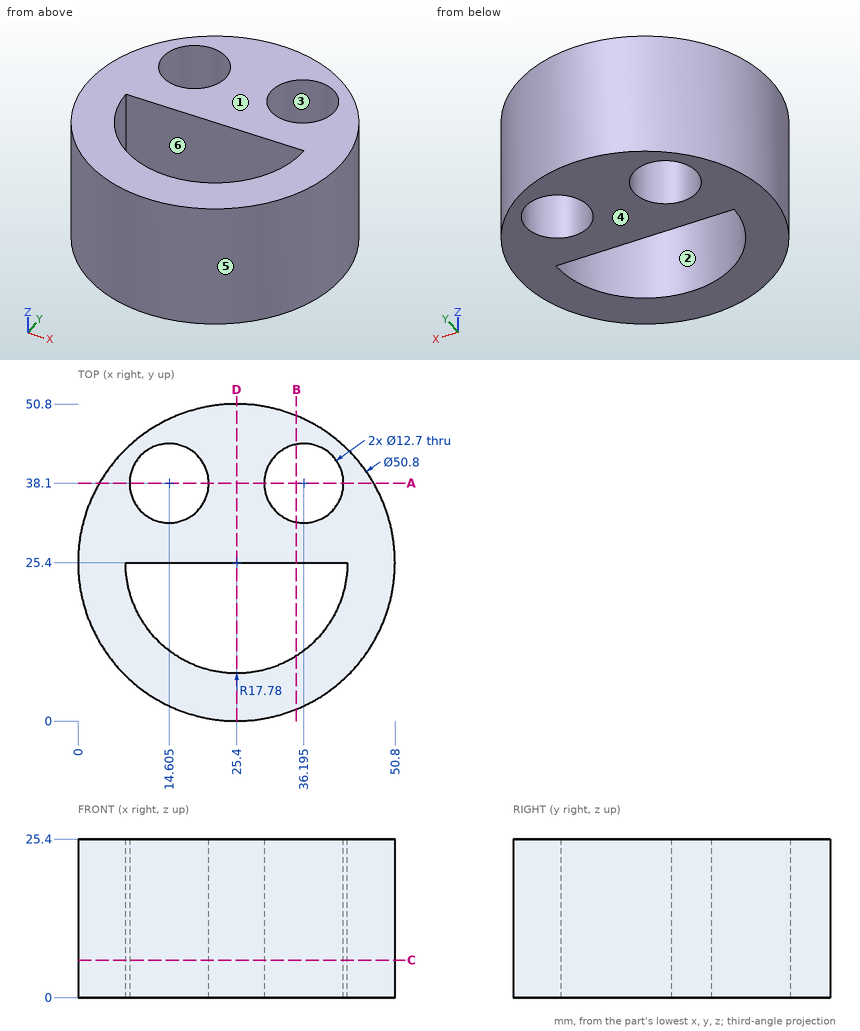
Verification items for this drawing (mm, ordinates from the low corner). A direction names the side the tool comes from. Coordinates: 2 decimals unless noted, no trailing zeros. Loops run counter-clockwise (first coordinate to the right, second up) from the corner with the lowest first, then second, coordinate; pieces in that order, holes last.
Item 1: Sectioned sample at B-B, the plane x = 35. Record the boundary of the cut face in (y, z).
Item 2: Release check for a two-part mould opening along Y. For the marked faces 3, 4, 5 and 6 record: released by +Y, released by -Y, zero draft, split by the parting line, or undercut.
Item 3: Go/stop test with flat-tipped pins: pin 1 Ø7.5 at (x, z) = (18, 7.5) entering from -Y; pin 2 Ø6 at (x, z) = (13.5, 8) entering from -Y; pin 3 Ø10 at (y, z) = (13, 21) entering from +X. Record where each tip stops, or that it passes through.
Item 4: Sectioned sample at D-D, the plane x = 25.4. Record the boundary of the cut face in (y, z), then the cut area to 3 significant figures.
Item 5: Thickness scan on line 1 (Y direction, x = 38, z = 4.25); line 2 (Y direction, x = 16, z = 8.5); line 3 (X direction, y = 37.5, z = 2.5). Record the ranges inside material, lowest first.
Item 6: Access from +Z, -Z, +X, -X, +Y, -Y to the whole of each face (thin tool, end or side, straight path). Record for the marked faces 1 and 2.
Item 7: Sectioned sample at A-A, the plane y = 38.1. Record the boundary of the cut face in (x, z) (3 decimals), then the cut area to 3 significant figures.
Item 8: Sectioned sample at C-C, the plane z = 6. Record the boundary of the cut face in (x, y) (3 decimals).
Check result:
1. outline: (1.88, 0) - (10.43, 0) - (10.43, 25.4) - (1.88, 25.4) - close; (25.4, 0) - (31.86, 0) - (31.86, 25.4) - (25.4, 25.4) - close; (44.34, 0) - (48.92, 0) - (48.92, 25.4) - (44.34, 25.4) - close
2. face 3: undercut
2. face 4: zero draft
2. face 5: split by the parting line
2. face 6: undercut
3. pin 1: stops at y = 0.26
3. pin 2: stops at y = 1.61
3. pin 3: stops at x = 49.7
4. outline: (0, 0) - (7.62, 0) - (7.62, 25.4) - (0, 25.4) - close; (25.4, 0) - (50.8, 0) - (50.8, 25.4) - (25.4, 25.4) - close
4. area: 839 mm2
5. line 1: y = 3.35 to 12.86, 25.4 to 32.01, 44.19 to 47.45
5. line 2: y = 1.8 to 10.31, 25.4 to 31.91, 44.29 to 49
5. line 3: x = 3.07 to 8.28, 20.93 to 29.87, 42.52 to 47.73
6. face 1: +Z, +X, -X, +Y, -Y
6. face 2: +Z, -Z
7. outline: (3.403, 0) - (8.255, 0) - (8.255, 25.4) - (3.403, 25.4) - close; (20.955, 0) - (29.845, 0) - (29.845, 25.4) - (20.955, 25.4) - close; (42.545, 0) - (47.397, 0) - (47.397, 25.4) - (42.545, 25.4) - close
7. area: 472 mm2
8. outline: circle Ø50.8 at (25.4, 25.4); hole (7.62, 25.4) arc R17.78 ccw to (43.18, 25.4) - close; hole circle Ø12.7 at (14.605, 38.1); hole circle Ø12.7 at (36.195, 38.1)
